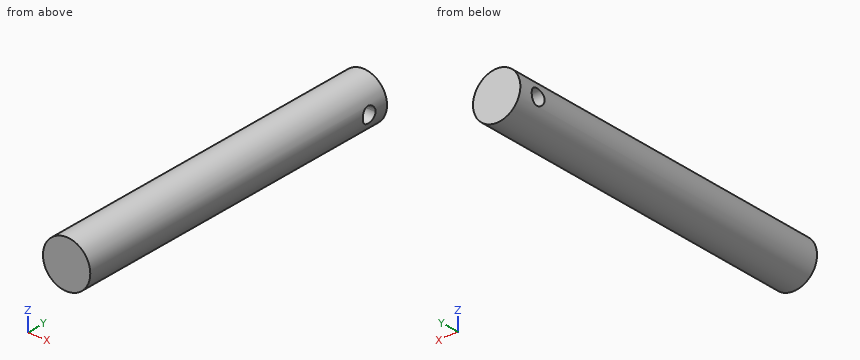
from build123d import *

# Parameters (mm, degrees)
F0_R     = 10
F1_DEPTH = 150
F4_D     = 6.5
F4_DEPTH = 10.001
F5_D     = 6.5


# Not quite as in the source:
# - a feature names something its author has since deleted; it is built from what else it names


with BuildPart() as f1:
    # F0 (on Front) → F1 (new body)
    with BuildSketch(Plane.XZ):
        Circle(F0_R)
    extrude(amount=F1_DEPTH)

    # F4 (through all, one way)
    with BuildSketch(Plane(origin=(0, 0, 0), x_dir=(0, 1, 0), z_dir=(-1, 0, 0))):
        with Locations((-9, 0)):
            Circle(F4_D / 2)
    extrude(amount=-F4_DEPTH, mode=Mode.SUBTRACT)

    # F5 (through all)
    with Locations(Plane.YZ):
        with Locations((-9, 0)):
            Hole(F5_D / 2)


solid = f1.part
For this review, take the finished solid that the model builds, in its own axes (mm). Give positions to 0.01 mm unless a question says otherwise; leave off trailing zeros. Loops run counter-clockwise (first coordinate to the right, second up) from the corner with the lowest first, then second, coordinate; pieces in that order, holes last. Notation, with made-up numbers: M 26.5,-27 L 50.5,-27 A29 cw 50.5,-3 Z; hole C -28.75,65.25 d8. An arc over 180 degrees is marked long. Answer as a JSON object with one key per item and string values. Group by question number.
Q1. Add section C-C on y = -9. Give the boundary of the cut face in (x, z).
Q2. For probe 1 along Y at (x, z) = (-1.5, 0); probe 2 along Z at (x, y) = (-4.25, -9); probe 3 along Y at (x, z) = (-8.25, 1.75), list the stretches that pass through material, from the lowest coordinate up. Write a range as [from, to].
Q3. Add section A-A on x = 4. Give the boundary of the cut face in (y, z).
Q4. Insertion check: P1, Ø12, axis at x = 6.5, y = -92.5, coming from the -Z side; P2, Ø4, axis at y = -110, z = 5, coming from the -X side. Each pin has a flat end and moves straight along its axis. Give the tip position at first contact, or say it passes through.
Q5. Add section B-B on y = -101. Give the boundary of the cut face in (x, z), and give its area (3 significant figures).
Q6. Add section D-D on z = -6. Give the boundary of the cut face in (x, y), and give its area (3 significant figures).
Checked values:
{
 "1": {"outline": "M -9.46,-3.25 A10 ccw 9.46,-3.25 Z; M -9.46,3.25 L 9.46,3.25 A10 ccw Z"},
 "2": {"probe 1": "[-150, -12.25], [-5.75, 0]", "probe 2": "[-9.05, -3.25], [3.25, 9.05]", "probe 3": "[-150, -11.74], [-6.26, 0]"},
 "3": {"outline": "M -150,-9.17 L 0,-9.17 L 0,9.17 L -150,9.17 Z; hole C -9,0 d6.5"},
 "4": {"P1": "z = -9.99", "P2": "x = -9.54"},
 "5": {"outline": "C 0,0 d20", "area": "314 mm²"},
 "6": {"outline": "M -8,-150 L 8,-150 L 8,0 L -8,0 Z", "area": "2,400 mm²"}
}
